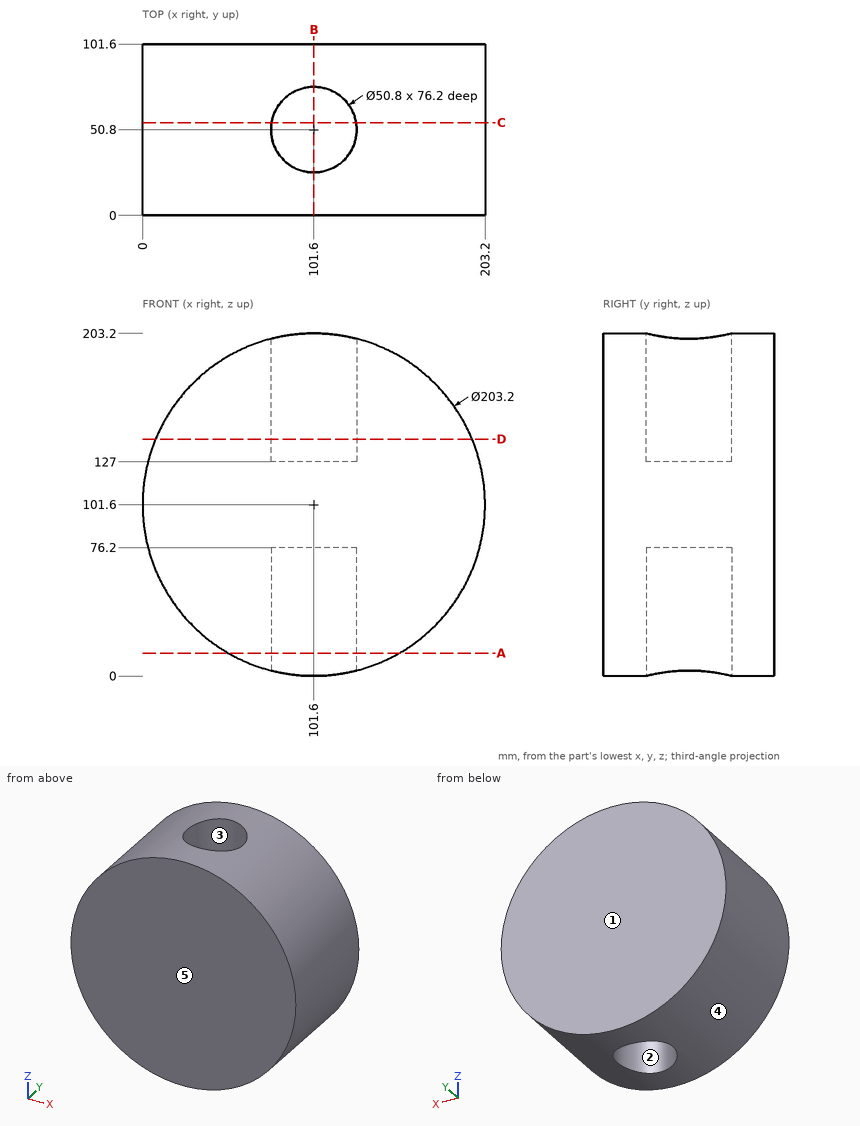
Drawing for the job (mm, zero at the part's lowest x, y, z). A direction names the side the tool comes from. Give positions to 0.01 mm unless a question says otherwise; leave off trailing zeros. Loops run counter-clockwise (first coordinate to the right, second up) from the corner with the lowest first, then second, coordinate; pieces in that order, holes last.
(1) Pin check, flat tips, straight feed: pin 1 (2 mm diameter, centred on y = 67, z = 123, fed in from +X); pin 2 (4 mm diameter, centred on x = 95.5, y = 13.5, fed in from -Z); pin 3 (6 mm diameter, centred on y = 43, z = 89, fed in from +X). Stop position of each tip, or through.
Return value:
pin 1: stops at x = 201.13
pin 2: stops at z = 0.08
pin 3: stops at x = 202.75
(2) Band-saw the part on A-A (z = 13.5). Write the cut outline in (x, y), and give its area (3 significant figures).
Return value:
outline: (50.99, 0) - (152.21, 0) - (152.21, 101.6) - (50.99, 101.6) - close; hole circle Ø50.8 at (101.6, 50.8)
area: 8,260 mm2
(3) 3-axis set-ups, long thin cutter, end or side, ignore diameter. For the marked faces 1 and 2: which of +Z, -Z, +X, -X, +Y, -Y reach the whole face in a straight line?
Return value:
face 1: +Z, -Z, +X, -X, +Y
face 2: -Z
(4) Drill centre lines: line 1 along Y through (x, z) = (101.6, 155.5); line 2 along X through (y, z) = (69, 173); line 3 along Z through (x, y) = (114.5, 60). Where is each one in solid material? Low to high.
Return value:
line 1: y = 0 to 25.4, 76.2 to 101.6
line 2: x = 29.32 to 83.88, 119.32 to 173.88
line 3: z = 76.2 to 127
(5) Band-saw the part on B-B (x = 101.6). Write the cut outline in (y, z).
Return value:
outline: (0, 0) - (25.4, 0) - (25.4, 76.2) - (76.2, 76.2) - (76.2, 0) - (101.6, 0) - (101.6, 203.2) - (76.2, 203.2) - (76.2, 127) - (25.4, 127) - (25.4, 203.2) - (0, 203.2) - close
(6) Band-saw the part on C-C (y = 55). Write the cut outline in (x, z).
Return value:
outline: (76.55, 3.14) - (76.55, 76.2) - (126.65, 76.2) - (126.65, 3.14) arc R101.6 ccw to (126.65, 200.06) - (126.65, 127) - (76.55, 127) - (76.55, 200.06) arc R101.6 ccw to start
(7) Band-saw the part on D-D (z = 140.5). Write the cut outline in (x, y).
Return value:
outline: (7.74, 0) - (195.46, 0) - (195.46, 101.6) - (7.74, 101.6) - close; hole circle Ø50.8 at (101.6, 50.8)
(8) Pull direction X, two halves, no side cores. Call the marked faces 3, 4 and 5: pulls with the +X half, pulls with the -X half, needs draft (parallel to the pull), parting line crosses it, or undercut.
Return value:
face 3: undercut
face 4: parting line crosses it
face 5: needs draft
